Input: part model. Units: mm. Frame: model coordinates. A direction names the side the tool comes from. Give positions to 0.01 mm unless a question says otherwise; leave off trailing zeros. Write each loop counter-clockwise with the first axis right and the second up, starting at its lowest first coordinate (ties: lowest second). Pieces come first, ordered by that corner, then holes. Notation, with made-up numbers: (28, 22.25) -> (47, 22.25) arc R17 cw to (47, 52.25) -> close; hole circle Ø2 at (-10.5, 3). An arc over 180 degrees is marked (long way). Answer as a JSON object with one key per item and string values. Group by question number.
from build123d import *

# Parameters (mm, degrees)
F0_W        = 15
F0_H        = 30
F1_DEPTH    = 48
F2_DEPTH    = 10
F3_W        = 15
F3_H        = 30
F4_DEPTH    = 38
F5_T1_DEPTH = 30


# Not quite as in the source:
# - a fillet or chamfer that OpenCascade refuses, or shapes differently, is made with other operations: its cross-section is extruded or revolved along the edge and cut away or added


with BuildPart() as f1:
    # F0 (on Top) → F1 (new body)
    with BuildSketch(Plane.XY):
        Polygon((21, 0), (0, 0), (-21, 0), (-21, 20), (-31, 20), (-31, -10), (31, -10), (31, 20), (21, 20), align=None)
        with Locations((38.5, 5)):
            Rectangle(F0_W, F0_H)
        with Locations((-38.5, 5)):
            Rectangle(F0_W, F0_H)
    extrude(amount=F1_DEPTH)

    # F0 (on Top) → F2 (join)
    with BuildSketch(Plane.XY):
        Polygon((46, -10), (31, -10), (-31, -10), (-46, -10), (-46, -28), (46, -28), align=None)
    extrude(amount=F2_DEPTH)

    # F3 (on face) → F4 (cut)
    with BuildSketch(Plane.XY.offset(48)):
        with Locations((-38.5, 5)):
            Rectangle(F3_W, F3_H)
        with Locations((38.5, 5)):
            Rectangle(F3_W, F3_H)
    extrude(amount=-F4_DEPTH, mode=Mode.SUBTRACT)

    # F5: fillet of radius 25 on 2 edges, made by hand

    # F5_s2 → F5_t1 (join)
    with BuildSketch(Plane.XZ.offset(-20)):
        with BuildLine():
            ThreePointArc((46, 10), (35.0834993366, 19.2198145372), (31, 32.9128784748))
            Line((31, 32.9128784748), (31, 10))
            Line((31, 10), (46, 10))
        make_face()
        with BuildLine():
            ThreePointArc((-46, 10), (-35.0834993366, 19.2198145372), (-31, 32.9128784748))
            Line((-31, 32.9128784748), (-31, 10))
            Line((-31, 10), (-46, 10))
        make_face()
    extrude(amount=F5_T1_DEPTH)


solid = f1.part
1. Section C-C (x = 0). Return the cut outline in (y, z), plus the area to 3 significant figures.
2. Section D-D (y = -4.5). Return the cut outline in (x, z), plus the area to 3 significant figures.
3. Reachability of faces 1 (the face through (-46, -4, 5)), 2 (the face through (0, 0, 24)), 3 (the face through (-1, -10, 29)), 4 (the face through (-1, -28, 5)), 5 (the face through (-31, 5, 41)) from +Z, -Z, +X, -X, +Y, -Y: full face, straight path, thin tool, end or side. Return the list, or none.
4. Contact query for flat-ended pins moving along their axis: pin 1 Ø14.5 at (x, y) = (-10, -23) entering from +Z; pin 2 Ø4.5 at (y, z) = (1.5, 43) entering from -X; pin 3 Ø6 at (y, z) = (11, 28.5) entering from -X. Output: stop coordinate, or through.
5. Section A-A (y = 10). Return the cut outline in (x, z).
6. Section B-B (z = 6.5). Return the cut outline in (x, y), plus the area to 3 significant figures.
7. Mould query, pull axis X, two halves, no side actions, for faces 6 (the face through (-21, 10, 24)), 7 (the face through (-1, -19, 10)), 8 (the face through (31, 5, 41)). Classes: pulls with the +X half, pulls with the -X half, needs draft (parallel to the pull), parting line crosses it, or undercut.
8. Line query: line 1 (X direction, y = 17, z = 41); line 2 (Y direction, x = 0.5, z = 4); line 3 (Y direction, x = 0, z = 36). Output: solid intervals per line, ascending.
Working result:
{
 "1": {"outline": "(-28, 0) -> (0, 0) -> (0, 48) -> (-10, 48) -> (-10, 10) -> (-28, 10) -> close", "area": "660 mm^2"},
 "2": {"outline": "(-46, 0) -> (46, 0) -> (46, 10) arc R25 cw to (31, 32.91) -> (31, 48) -> (-31, 48) -> (-31, 32.91) arc R25 cw to (-46, 10) -> close", "area": "3,470 mm^2"},
 "3": {"face 1": "+Z, -Z, -X, +Y, -Y", "face 2": "+Z, -Z, +Y", "face 3": "+Z, +X, -X, -Y", "face 4": "+Z, -Z, +X, -X, -Y", "face 5": "+Z, -X, +Y, -Y"},
 "4": {"pin 1": "stops at z = 10", "pin 2": "stops at x = -31", "pin 3": "stops at x = -32.12"},
 "5": {"outline": "(-46, 0) -> (-21, 0) -> (-21, 48) -> (-31, 48) -> (-31, 32.91) arc R25 cw to (-46, 10) -> close; (21, 0) -> (46, 0) -> (46, 10) arc R25 cw to (31, 32.91) -> (31, 48) -> (21, 48) -> close"},
 "6": {"outline": "(-46, -28) -> (46, -28) -> (46, 20) -> (21, 20) -> (21, 0) -> (-21, 0) -> (-21, 20) -> (-46, 20) -> close", "area": "3,580 mm^2"},
 "7": {"face 6": "undercut", "face 7": "needs draft", "face 8": "pulls with the +X half"},
 "8": {"line 1": "x = -31 to -21, 21 to 31", "line 2": "y = -28 to 0", "line 3": "y = -10 to 0"}
}
